Input: part model. Units: mm. Frame: model coordinates. Round coordinates to 2 decimals unless told otherwise and drop trailing zeros. Loops run counter-clockwise (first coordinate to the right, second up) from the corner with the lowest first, then second, coordinate; pieces in that order, holes last. Notation, with made-up numbers: (46, 32.5) -> (66, 32.5) arc R10 cw to (66, 38.5) -> close; hole circle Ø4 at (28, -8). An arc over 180 degrees is marked (long way). Answer as a JSON object with one key per item and string values.
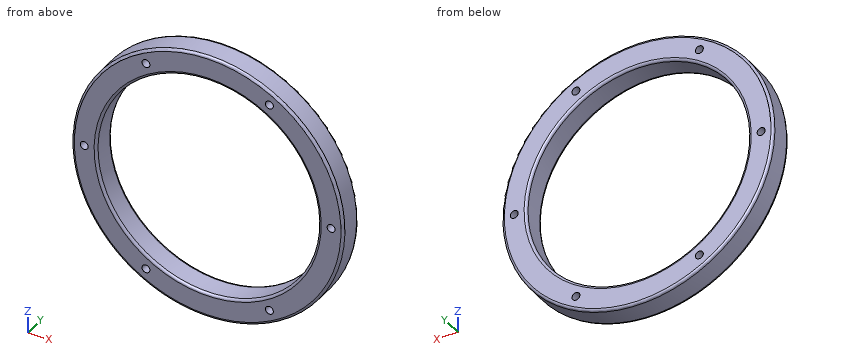
```python
from build123d import *

# Parameters (mm, degrees)
SKETCH_1_R      = 55
SKETCH_1_R_2    = 45
SKETCH_1_R_3    = 1.6
EXTRUDE_1_DEPTH = 10
FILLET_1_R      = 1


with BuildPart() as part:
    # 草图1 → 凸台-拉伸1 (new body)
    with BuildSketch(Plane(origin=(0, 0, 0), x_dir=(1, 0, 0), z_dir=(0, 1, 0))):
        with Locations(Location((0, 0, 0), (0, 0, 270))):
            Circle(SKETCH_1_R)
        with Locations(Location((0, 0, 0), (0, 0, 270))):
            Circle(SKETCH_1_R_2, mode=Mode.SUBTRACT)
        with Locations(Location((50, 0, 0), (0, 0, 270))):
            Circle(SKETCH_1_R_3, mode=Mode.SUBTRACT)
        with Locations(Location((25, -43.301270189, 0), (0, 0, 270))):
            Circle(SKETCH_1_R_3, mode=Mode.SUBTRACT)
        with Locations(Location((-25, -43.301270189, 0), (0, 0, 270))):
            Circle(SKETCH_1_R_3, mode=Mode.SUBTRACT)
        with Locations(Location((-50, 0, 0), (0, 0, 270))):
            Circle(SKETCH_1_R_3, mode=Mode.SUBTRACT)
        with Locations(Location((-25, 43.301270189, 0), (0, 0, 270))):
            Circle(SKETCH_1_R_3, mode=Mode.SUBTRACT)
        with Locations(Location((25, 43.301270189, 0), (0, 0, 270))):
            Circle(SKETCH_1_R_3, mode=Mode.SUBTRACT)
    extrude(amount=EXTRUDE_1_DEPTH)

    # 圆角1
    fillet_1_edges = [part.edges().sort_by_distance(p)[0] for p in [
        (0, 0, -55),
        (0, 10, -55),
        (0, 0, -45),
        (0, 10, -45),
    ]]
    fillet(fillet_1_edges, radius=FILLET_1_R)


solid = part.part
```
1) Contact query for flat-ended pins moving along their axis: P1, Ø5, axis at y = 6.5, z = -36.5, coming from the -X side; P2, Ø4, axis at y = 3, z = -40.5, coming from the +X side; P3, Ø5, axis at x = -50, z = 0, coming from the +Y side; P4, Ø2, axis at y = 1.5, z = 36.5, coming from the +X side. Output: stop coordinate, or through.
Output:
{"P1": "stops at x = -43.23", "P2": "stops at x = 39.28", "P3": "stops at y = 10", "P4": "stops at x = 42.01"}
2) Ray query, probe 1 along X at (y, z) = (8.25, 0); probe 2 along Z at (x, y) = (-29.5, 8); probe 3 along X at (y, z) = (2, -31). Return the intervals inside material, ascending.
Output:
{"probe 1": "x = -55 to -51.6, -48.4 to -45, 45 to 48.4, 51.6 to 55", "probe 2": "z = -46.42 to -33.98, 33.98 to 46.42", "probe 3": "x = -45.43 to -32.62, 32.62 to 45.43"}
3) Section B-B, the plane y = 7.75. Output: boundary loops of the cut face in (x, z), plus the area to 3 significant figures.
Output:
{"outline": "circle Ø110 at (0, 0); hole circle Ø3.2 at (-50, 0); hole circle Ø90 at (0, 0); hole circle Ø3.2 at (-25, -43.3); hole circle Ø3.2 at (-25, 43.3); hole circle Ø3.2 at (25, -43.3); hole circle Ø3.2 at (25, 43.3); hole circle Ø3.2 at (50, 0)", "area": "3,090 mm^2"}
4) Section A-A, the plane x = 0. Output: boundary loops of the cut face in (y, z).
Output:
{"outline": "(0, -54) arc R1 ccw to (1, -55) -> (9, -55) arc R1 ccw to (10, -54) -> (10, -46) arc R1 ccw to (9, -45) -> (1, -45) arc R1 ccw to (0, -46) -> close; (0, 46) arc R1 ccw to (1, 45) -> (9, 45) arc R1 ccw to (10, 46) -> (10, 54) arc R1 ccw to (9, 55) -> (1, 55) arc R1 ccw to (0, 54) -> close"}
5) Section C-C, the plane z = -43. Count the separate pieces of the cut face and the enclosed holes in it, plus the area to 3 significant figures.
Output:
{"separate pieces": "4", "enclosed holes": "0", "area": "354 mm^2"}
